```python
from build123d import *

# Parameters (mm, degrees)
CYLINDER018_R     = 1
CYLINDER018_DEPTH = 26
CYLINDER019_R     = 1
CYLINDER019_DEPTH = 26
BOX007_W          = 30
BOX007_H          = 2
BOX007_DEPTH      = 26
CYLINDER016_R     = 2.5
CYLINDER016_DEPTH = 10
CYLINDER017_R     = 2.5
CYLINDER017_DEPTH = 10
BOX005_W          = 15
BOX005_H          = 34
BOX005_DEPTH      = 2
BOX004_W          = 1.6
BOX004_H          = 20
BOX004_DEPTH      = 26
CYLINDER010_R     = 11
CYLINDER010_DEPTH = 22
CYLINDER009_R     = 30.5
CYLINDER009_DEPTH = 22
CYLINDER008_R     = 9
CYLINDER008_DEPTH = 26
CYLINDER007_R     = 30.5
CYLINDER007_DEPTH = 26


with BuildPart() as cylinder018:
    # Cylinder018 → Cylinder018 (new body)
    with BuildSketch(Plane(origin=(39.5, 17, 0), x_dir=(1, 0, 0), z_dir=(0, 0, 1))):
        Circle(CYLINDER018_R)
    extrude(amount=CYLINDER018_DEPTH)


with BuildPart() as wireholes:
    # Cylinder019 → Cylinder019 (new body)
    with BuildSketch(Plane(origin=(23, 17, 0), x_dir=(1, 0, 0), z_dir=(0, 0, 1))):
        Circle(CYLINDER019_R)
    extrude(amount=CYLINDER019_DEPTH)

    # Fusion007: union Cylinder018
    add(cylinder018.part)


with BuildPart() as cube007:
    # Box007 → Box007 (new body)
    with BuildSketch(Plane(origin=(53, 16, 0), x_dir=(1, 0, 0), z_dir=(0, 0, 1))):
        with Locations((15, 1)):
            Rectangle(BOX007_W, BOX007_H)
    extrude(amount=BOX007_DEPTH)


with BuildPart() as cylinder016:
    # Cylinder016 → Cylinder016 (new body)
    with BuildSketch(Plane(origin=(20, 5, 0), x_dir=(1, 0, 0), z_dir=(0, 0, 1))):
        Circle(CYLINDER016_R)
    extrude(amount=CYLINDER016_DEPTH)


with BuildPart() as obj1:
    # Cylinder017 → Cylinder017 (new body)
    with BuildSketch(Plane(origin=(20, 29, 0), x_dir=(1, 0, 0), z_dir=(0, 0, 1))):
        Circle(CYLINDER017_R)
    extrude(amount=CYLINDER017_DEPTH)

    # Fusion005: union Cylinder016
    add(cylinder016.part)


with BuildPart() as cut010:
    # Box005 → Box005 (new body)
    with BuildSketch(Plane(origin=(15, 0, 0), x_dir=(1, 0, 0), z_dir=(0, 0, 1))):
        with Locations((7.5, 17)):
            Rectangle(BOX005_W, BOX005_H)
    extrude(amount=BOX005_DEPTH)

    # Cut010: cut obj1
    add(obj1.part, mode=Mode.SUBTRACT)


with BuildPart() as cube004:
    # Box004 → Box004 (new body)
    with BuildSketch(Plane(origin=(49.9, 7, 0), x_dir=(1, 0, 0), z_dir=(0, 0, 1))):
        with Locations((0.8, 10)):
            Rectangle(BOX004_W, BOX004_H)
    extrude(amount=BOX004_DEPTH)


with BuildPart() as cylinder010:
    # Cylinder010 → Cylinder010 (new body)
    with BuildSketch(Plane.XY):
        Circle(CYLINDER010_R)
    extrude(amount=CYLINDER010_DEPTH)


with BuildPart() as obj2:
    # Cylinder009 → Cylinder009 (new body)
    with BuildSketch(Plane.XY):
        Circle(CYLINDER009_R)
    extrude(amount=CYLINDER009_DEPTH)

    # Cut004: cut Cylinder010
    add(cylinder010.part, mode=Mode.SUBTRACT)


with BuildPart() as obj2_1:
    # Cut004 placement: moved
    add(obj2.part.moved(Location((51.5, 17, 2))))


with BuildPart() as cylinder008:
    # Cylinder008 → Cylinder008 (new body)
    with BuildSketch(Plane.XY):
        Circle(CYLINDER008_R)
    extrude(amount=CYLINDER008_DEPTH)


with BuildPart() as coilholder:
    # Cylinder007 → Cylinder007 (new body)
    with BuildSketch(Plane.XY):
        Circle(CYLINDER007_R)
    extrude(amount=CYLINDER007_DEPTH)

    # Cut002: cut Cylinder008
    add(cylinder008.part, mode=Mode.SUBTRACT)


with BuildPart() as coilholder_1:
    # Cut002 placement: moved
    add(coilholder.part.moved(Location((51.5, 17, 0))))

    # Cut005: cut obj2
    add(obj2_1.part, mode=Mode.SUBTRACT)

    # Cut007: cut Cube004
    add(cube004.part, mode=Mode.SUBTRACT)

    # Fusion006: union Cut010
    add(cut010.part)

    # Cut012: cut Cube007
    add(cube007.part, mode=Mode.SUBTRACT)

    # Cut013: cut WireHoles
    add(wireholes.part, mode=Mode.SUBTRACT)


solid = coilholder_1.part
```
Could you check a few things on this model? Use its own coordinates, in mm. A direction names the side the tool comes from. Coordinates: 2 decimals unless noted, no trailing zeros. Write each loop counter-clockwise with the first axis right and the second up, starting at its lowest first coordinate (ties: lowest second). Pieces come first, ordered by that corner, then holes. Notation, with made-up numbers: (72, -16) -> (110, -16) arc R11 ccw to (110, -12) -> close; hole circle Ø2 at (58, -28.75). An arc over 180 degrees is marked (long way). One line per question, with ' | ' between items. Start each with the question number.
1. Will these pins go through, and if not, where does the flat tip stop? P1, Ø4.5, axis at x = 20, y = 29, coming from the -Z side; P2, Ø0.5, axis at x = 51, z = 8.5, coming from the +Y side; P3, Ø0.5, axis at y = 26.5, z = 9, coming from the -X side; P4, Ø1.8, axis at x = 50.5, z = 12, coming from the -Y side.
2. For faces 4 (the face through (21, 34, 1)), 5 (the face through (62, 16, 13)), 6 (the face through (57.568, 23.647, 12.818)), which set-ups out of +Z, -Z, +X, -X, +Y, -Y let a thin tool reach every point of the face, with its end or its side?
3. If we section it at B-B (y = 5): Please give me the cut outline in (x, z).
4. Thinking about a two-plate mould opening in X: for faces 1 (the face through (23, 16, 1)), 2 (the face through (40.51, 17.47, 12.85)), 3 (the face through (21, 0, 1)), which applies, pulls with the +X half, pulls with the -X half, needs draft (parallel to the pull), parting line crosses it, or undercut?
5. If we section it at D-D (z = 13): Please give me the cut outline in (x, y), and give its area (3 significant figures).
6. Please list where these lines run through material, in increasing order: line 1 along X through (y, z) = (17, 1); line 2 along Y through (x, z) = (20, 1.6); line 3 along Z through (x, y) = (52, 0.5).
7. If we section it at C-C (x = 20): Please give me the cut outline in (y, z).
8. If we section it at A-A (x = 69): Please give me the cut outline in (y, z), and give its area (3 significant figures).
Return value:
1) P1: passes through | P2: stops at y = 28 | P3: stops at x = 45.55 | P4: stops at y = 6
2) face 4: +Z, -Z, -X, +Y | face 5: +Z, -Z, +X | face 6: +Z, -Z
3) outline: (15, 0) -> (17.5, 0) -> (17.5, 2) -> (15, 2) -> close; (22.5, 0) -> (79.54, 0) -> (79.54, 2) -> (22.5, 2) -> close; (23.46, 24) -> (79.54, 24) -> (79.54, 26) -> (23.46, 26) -> close
4) face 1: undercut | face 2: parting line crosses it | face 3: needs draft
5) outline: (49.9, 7) -> (49.9, 8.14) arc R9 cw to (49.9, 25.86) -> (49.9, 27) -> (51.5, 27) -> (51.5, 26) arc R9 cw to (60.44, 18) -> (62.45, 18) arc R11 ccw (long way) to (62.45, 16) -> (60.44, 16) arc R9 cw to (51.5, 8) -> (51.5, 7) -> close | area: 118 mm²
6) line 1: x = 15 to 22, 24 to 38.5, 40.5 to 42.5 | line 2: y = 0 to 2.5, 7.5 to 26.5, 31.5 to 34 | line 3: z = 0 to 2, 24 to 26
7) outline: (0, 0) -> (2.5, 0) -> (2.5, 2) -> (0, 2) -> close; (7.5, 0) -> (26.5, 0) -> (26.5, 2) -> (7.5, 2) -> close; (31.5, 0) -> (34, 0) -> (34, 2) -> (31.5, 2) -> close
8) outline: (-7.98, 0) -> (16, 0) -> (16, 2) -> (-7.98, 2) -> close; (-7.98, 24) -> (16, 24) -> (16, 26) -> (-7.98, 26) -> close; (18, 0) -> (41.98, 0) -> (41.98, 2) -> (18, 2) -> close; (18, 24) -> (41.98, 24) -> (41.98, 26) -> (18, 26) -> close | area: 192 mm²
